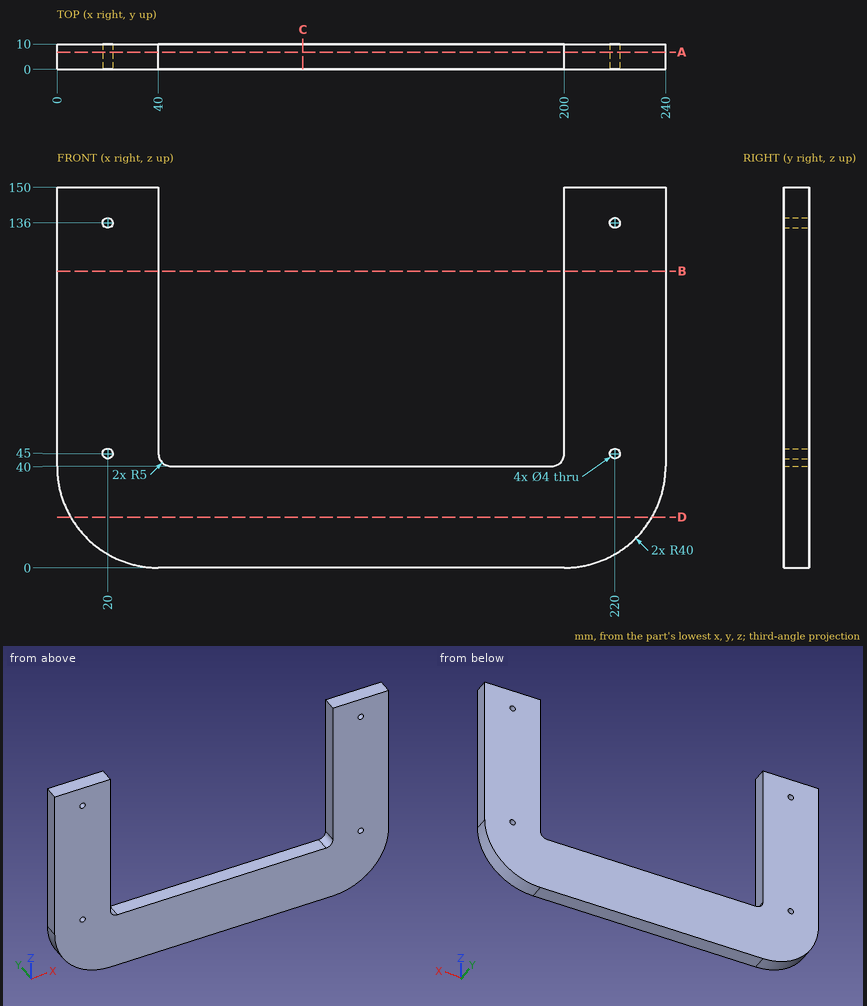
Verification items for this drawing (mm, ordinates from the low corner). Give positions to 0.01 mm unless a question says otherwise; leave off trailing zeros. Write each loop counter-clockwise with the first axis right and the second up, starting at its lowest first coordinate (ties: lowest second). Pieces come first, ordered by that corner, then holes.
1) Cross-section at D-D (z = 20). Record the boundary of the cut face in (x, y).
Values follow:
outline: (5.36, 0) - (234.64, 0) - (234.64, 10) - (5.36, 10) - close
2) Cross-section at B-B (z = 117). Record the boundary of the cut face in (x, y), plus the area to 3 significant figures.
Values follow:
outline: (0, 0) - (40, 0) - (40, 10) - (0, 10) - close; (200, 0) - (240, 0) - (240, 10) - (200, 10) - close
area: 800 mm2
3) Cross-section at A-A (y = 6.75). Record the boundary of the cut face in (x, z).
Values follow:
outline: (0, 40) arc R40 ccw to (40, 0) - (200, 0) arc R40 ccw to (240, 40) - (240, 150) - (200, 150) - (200, 45) arc R5 cw to (195, 40) - (45, 40) arc R5 cw to (40, 45) - (40, 150) - (0, 150) - close; hole circle Ø4 at (20, 45); hole circle Ø4 at (20, 136); hole circle Ø4 at (220, 45); hole circle Ø4 at (220, 136)
4) Thickness scan on line 1 (X direction, y = 7.5, z = 136); line 2 (Z direction, x = 220, y = 4); line 3 (X direction, y = 9.75, z = 107). Record the ranges inside material, lowest first.
Values follow:
line 1: x = 0 to 18, 22 to 40, 200 to 218, 222 to 240
line 2: z = 5.36 to 43, 47 to 134, 138 to 150
line 3: x = 0 to 40, 200 to 240
5) Cross-section at C-C (x = 97). Record the boundary of the cut face in (y, z).
Values follow:
outline: (0, 0) - (10, 0) - (10, 40) - (0, 40) - close
6) Go/stop test with flat-tipped pins: pin 1 Ø10 at (x, z) = (190.5, 102.5) entering from -Y; pin 2 Ø6.5 at (x, z) = (220, 45) entering from +Y; pin 3 Ø3 at (x, y) = (103, 7) entering from +Z. Record where each tip stops, or that it passes through.
Values follow:
pin 1: passes through
pin 2: stops at y = 10
pin 3: stops at z = 40
